Autodesk Inventor part; units mm, degrees
ref_plane "SCHRAUBE_XY" through (0, 0, 0) normal (-1, 0, 0) x (0, 0, -1)
ref_plane "SCHRAUBE_YZ" through (0, 0, 0) normal (0, 0, -1) x (0, -1, 0)
ref_plane "SCHRAUBE_ZX" through (0, 0, 0) normal (0, -1, 0) x (-1, 0, 0)
sketch "Sketch_1" plane through (0, 0, 0) normal (0, 0, 1) x (1, 0, 0)
  line L0 (12, 0) -> (-3.6, 0)
  line L1 (-3.6, 0) -> (-3.6, 2.6)
  arc A0 (-1.6, 5) -> (-3.6, 2.6) centre (-0.2671, 1.8559) ccw
  line L2 (-1.6, 5) -> (-1.6, 5.45)
  arc A1 (-1.3, 5.75) -> (-1.6, 5.45) centre (-1.3, 5.45) ccw
  line L3 (-1.3, 5.75) -> (-0.425, 5.75)
  arc A2 (0, 5.325) -> (-0.425, 5.75) centre (-0.425, 5.325) ccw
  line L4 (0, 5.325) -> (0, 2.5)
  line L5 (0, 2.5) -> (8.6241, 2.5)
  line L6 (8.6241, 2.5) -> (12, 1.5)
  line L7 (12, 1.5) -> (12, 0)
  line L8 (12, 0) -> (-3.6, 0)
revolve "Revolution1" add sketch "Sketch_1" angle 360 about axis through (12, 0, 0) along (1, 0, 0)
ref_plane "SCHRAUBE_XY" through (0, 0, 0) normal (-1, 0, 0) x (0, 0, -1)
ref_plane "SCHRAUBE_YZ" through (0, 0, 0) normal (0, 0, -1) x (0, -1, 0)
ref_plane "SCHRAUBE_ZX" through (0, 0, 0) normal (0, -1, 0) x (-1, 0, 0)
properties part number "1301.000_10_(1)"
Geometry check sheet. Reference: the model listing, model coordinates, mm. A direction names the side the tool comes from. Round coordinates to 2 decimals unless told otherwise and drop trailing zeros. Order: outer loops, then holes, each group sorted by start corner. A loop starts at its lowest first (then second) coordinate and runs counter-clockwise, first axis right, second up. Notation, with made-up numbers: (18.5, 26) - (33.5, 26) arc R24 cw to (33.5, 52) - close; hole circle Ø7 at (-3, 20.25). An arc over 180 degrees is marked (long way). Use a Markdown table: item, result. Add a question column.
1) Thickness scan on line 1 along Z through (x, y) = (2, 2); line 2 along Z through (x, y) = (6, 1.5); line 3 along X through (y, z) = (-2.75, -4.75). Record the ranges inside material, lowest first.
2) Section check A-A (x = 3). Record the cut outline in (y, z), then the cut area to 3 significant figures.
3) Set-up check for faces 1 (the flat face through (0, -2.44, -1.11)), 2 (the flat face through (-3.6, 0, 0)): record each of +Z, -Z, +X, -X, +Y, -Y from which the full face is reachable in a straight line by a thin tool's end or side.
4) Gauge pin test, flat ends, axial feed: P1, Ø4, axis at x = 8, z = -1, coming from the +Y side; P2, Ø1.5, axis at x = 5.5, z = 0, coming from the -Y side; P3, Ø1.5, axis at x = 9, y = -2.5, coming from the -Z side. Record the tip position at first contact, or that the pin passes through.
Established:
| question | item | result |
|---|---|---|
| 1 | line 1 | -1.5 to 1.5 |
| 1 | line 2 | -2 to 2 |
| 1 | line 3 | -1.6 to -0.03 |
| 2 | outline | circle Ø5 at (0, 0) |
| 2 | area | 19.6 mm2 |
| 3 | face 1 | +X |
| 3 | face 2 | +Z, -Z, -X, +Y, -Y |
| 4 | P1 | y = 2.5 |
| 4 | P2 | y = -2.5 |
| 4 | P3 | z = -1.69 |
